Geometry: final body of the model. Coordinates: model frame, mm. Round coordinates to 2 decimals unless told otherwise and drop trailing zeros. Loops run counter-clockwise (first coordinate to the right, second up) from the corner with the lowest first, then second, coordinate; pieces in that order, holes last. Notation, with made-up numbers: (74.5, 25.5) - (119.5, 25.5) arc R33 ccw to (119.5, 54.5) - close; hole circle Ø7 at (52, -8.5). An arc over 180 degrees is marked (long way). Answer in a Markdown table with one row per item. Add a question column.
from build123d import *

# Parameters (mm, degrees)
BOSS_EXTRUDE1_DEPTH = 3048
SKETCH4_W           = 82.55
SKETCH4_H           = 485.775
CUT_EXTRUDE1_DEPTH  = 3049.558881053


with BuildPart() as part:
    # Sketch1 → Boss-Extrude1 (new body)
    with BuildSketch(Plane.XY):
        with BuildLine():
            Line((-36.22675, 20.6375), (-3.46075, 20.6375))
            ThreePointArc((-3.46075, 20.6375), (-1.013630207, 19.623869793), (0, 17.17675))
            Line((0, 17.17675), (0, -17.17675))
            ThreePointArc((0, -17.17675), (-1.013630207, -19.623869793), (-3.46075, -20.6375))
            Line((-3.46075, -20.6375), (-36.22675, -20.6375))
            ThreePointArc((-36.22675, -20.6375), (-39.796401808, -19.158901808), (-41.275, -15.58925))
            Line((-41.275, -15.58925), (-41.275, -14.57325))
            ThreePointArc((-41.275, -14.57325), (-40.261369793, -12.126130207), (-37.81425, -11.1125))
            Line((-37.81425, -11.1125), (-35.5346, -11.1125))
            ThreePointArc((-35.5346, -11.1125), (-34.1376, -12.5095), (-35.5346, -13.9065))
            Line((-35.5346, -13.9065), (-37.81425, -13.9065))
            ThreePointArc((-37.81425, -13.9065), (-38.285713446, -14.101786554), (-38.481, -14.57325))
            Line((-38.481, -14.57325), (-38.481, -15.58925))
            ThreePointArc((-38.481, -15.58925), (-37.820745461, -17.183245461), (-36.22675, -17.8435))
            Line((-36.22675, -17.8435), (-3.46075, -17.8435))
            ThreePointArc((-3.46075, -17.8435), (-2.989286554, -17.648213446), (-2.794, -17.17675))
            Line((-2.794, -17.17675), (-2.794, 17.17675))
            ThreePointArc((-2.794, 17.17675), (-2.989286554, 17.648213446), (-3.46075, 17.8435))
            Line((-3.46075, 17.8435), (-36.22675, 17.8435))
            ThreePointArc((-36.22675, 17.8435), (-37.820745461, 17.183245461), (-38.481, 15.58925))
            Line((-38.481, 15.58925), (-38.481, 14.57325))
            ThreePointArc((-38.481, 14.57325), (-38.285713446, 14.101786554), (-37.81425, 13.9065))
            Line((-37.81425, 13.9065), (-35.5346, 13.9065))
            ThreePointArc((-35.5346, 13.9065), (-34.1376, 12.5095), (-35.5346, 11.1125))
            Line((-35.5346, 11.1125), (-37.81425, 11.1125))
            ThreePointArc((-37.81425, 11.1125), (-40.261369793, 12.126130207), (-41.275, 14.57325))
            Line((-41.275, 14.57325), (-41.275, 15.58925))
            ThreePointArc((-41.275, 15.58925), (-39.796401808, 19.158901808), (-36.22675, 20.6375))
        make_face()
    extrude(amount=-BOSS_EXTRUDE1_DEPTH)


with BuildPart() as body_2:
    # Mirror1: mirrored copy
    add(part.part.mirror(Plane(origin=(0, 17.17675, -3048), x_dir=(0, 0, 1), z_dir=(1, 0, 0))))


with BuildPart() as cut_extrude1_tool:
    # Sketch4 → Cut-Extrude1 (new, through all)
    with BuildSketch(Plane.XZ.offset(20.6375)):
        with Locations((0, -242.8875)):
            Rectangle(SKETCH4_W, SKETCH4_H)
    extrude(amount=-CUT_EXTRUDE1_DEPTH)


with BuildPart() as part_1:
    add(part.part)

    # Cut-Extrude1: cut by cut_extrude1_tool
    add(cut_extrude1_tool.part, mode=Mode.SUBTRACT)


with BuildPart() as body_2_1:
    add(body_2.part)

    # Cut-Extrude1: cut by cut_extrude1_tool
    add(cut_extrude1_tool.part, mode=Mode.SUBTRACT)

    # Combine1: union part
    add(part_1.part)


solid = body_2_1.part
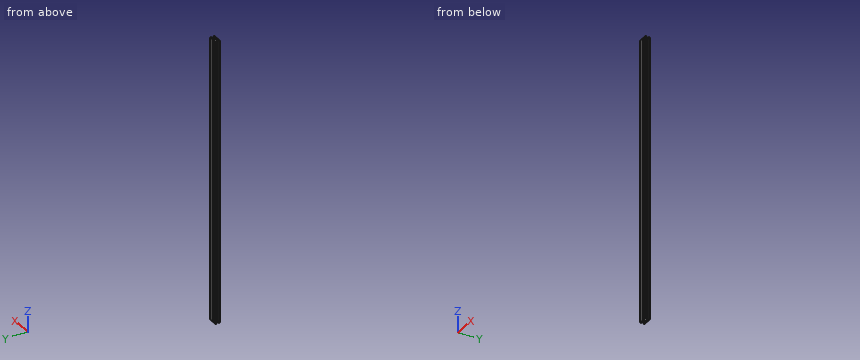
1) Contact query for flat-ended pins moving along their axis: pin 1 Ø3 at (y, z) = (-11.5, -1091.5) entering from +X; pin 2 Ø1.5 at (y, z) = (-4.5, -1742) entering from -X; pin 3 Ø2 at (y, z) = (9, -1916.5) entering from +X. Output: stop coordinate, or through.
2) Section A-A, the plane x = -18. Return the cut outline in (y, z) (1 decimal), and give its area (3 significant figures).
3) Material intervals for line 1 along X through (y, z) = (15, -956.5) (3 decimals); line 2 along Y through (x, z) = (38, -1098.5); line 3 along Y through (x, z) = (-37, -741.5), sorted ascending. Write a range as from..to.
Evaluation:
| question | item | result |
|---|---|---|
| 1 | pin 1 | stops at x = 40.9 |
| 1 | pin 2 | stops at x = -2.79 |
| 1 | pin 3 | stops at x = 2.79 |
| 2 | outline | (-20.6, -3048) - (-17.8, -3048) - (-17.8, -485.8) - (-20.6, -485.8) - close; (17.8, -3048) - (20.6, -3048) - (20.6, -485.8) - (17.8, -485.8) - close |
| 2 | area | 14,300 mm² |
| 3 | line 1 | x = -41.275..-38.481, -2.794..2.794, 38.481..41.275 |
| 3 | line 2 | y = -20.32..-16.98, -13.93..-11.12, 11.12..13.93, 16.98..20.32 |
| 3 | line 3 | y = -20.58..-17.71, -13.91..-11.11, 11.11..13.91, 17.71..20.58 |
